from build123d import *

# Parameters (mm, degrees)
SKETCH_1_W      = 220
SKETCH_1_H      = 220
SKETCH_1_R      = 2
SKETCH_1_R_2    = 1.6
SKETCH_1_W_2    = 5
SKETCH_1_H_2    = 20
SKETCH_1_W_3    = 10
SKETCH_1_H_3    = 5.002557866
SKETCH_1_H_4    = 5
EXTRUDE_1_DEPTH = 5


with BuildPart() as part:
    # 草图1 → 凸台-拉伸1 (new body)
    with BuildSketch(Plane(origin=(0, 0, 0), x_dir=(0, 0, -1), z_dir=(1, 0, 0))):
        with Locations((1.240063593, -23.177255758)):
            Rectangle(SKETCH_1_W, SKETCH_1_H)
        with Locations((-22.759936407, 7.822744242)):
            Circle(SKETCH_1_R, mode=Mode.SUBTRACT)
        with Locations((-40.759936407, 7.822744242)):
            Circle(SKETCH_1_R, mode=Mode.SUBTRACT)
        with Locations((-40.759936407, 31.822744242)):
            Circle(SKETCH_1_R, mode=Mode.SUBTRACT)
        with Locations((-22.759936407, 31.822744242)):
            Circle(SKETCH_1_R, mode=Mode.SUBTRACT)
        with Locations((-22.759936407, -78.177255758)):
            Circle(SKETCH_1_R, mode=Mode.SUBTRACT)
        with Locations((-40.759936407, -78.177255758)):
            Circle(SKETCH_1_R, mode=Mode.SUBTRACT)
        with Locations((-40.759936407, -54.177255758)):
            Circle(SKETCH_1_R, mode=Mode.SUBTRACT)
        with Locations((-22.759936407, -54.177255758)):
            Circle(SKETCH_1_R, mode=Mode.SUBTRACT)
        with Locations((43.240063593, 7.822744242)):
            Circle(SKETCH_1_R, mode=Mode.SUBTRACT)
        with Locations((25.240063593, 7.822744242)):
            Circle(SKETCH_1_R, mode=Mode.SUBTRACT)
        with Locations((25.240063593, 31.822744242)):
            Circle(SKETCH_1_R, mode=Mode.SUBTRACT)
        with Locations((43.240063593, 31.822744242)):
            Circle(SKETCH_1_R, mode=Mode.SUBTRACT)
        with Locations((43.240063593, -78.177255758)):
            Circle(SKETCH_1_R, mode=Mode.SUBTRACT)
        with Locations((25.240063593, -78.177255758)):
            Circle(SKETCH_1_R, mode=Mode.SUBTRACT)
        with Locations((25.240063593, -54.177255758)):
            Circle(SKETCH_1_R, mode=Mode.SUBTRACT)
        with Locations((43.240063593, -54.177255758)):
            Circle(SKETCH_1_R, mode=Mode.SUBTRACT)
        with Locations((105.740063593, 81.322744242)):
            Circle(SKETCH_1_R_2, mode=Mode.SUBTRACT)
        with Locations((-103.259936407, 81.322744242)):
            Circle(SKETCH_1_R_2, mode=Mode.SUBTRACT)
        with Locations((-103.259936407, -127.677255758)):
            Circle(SKETCH_1_R_2, mode=Mode.SUBTRACT)
        with Locations((105.740063593, -127.677255758)):
            Circle(SKETCH_1_R_2, mode=Mode.SUBTRACT)
        with Locations((13.740063593, -23.177255758)):
            Rectangle(SKETCH_1_W_2, SKETCH_1_H_2, mode=Mode.SUBTRACT)
        with Locations((-11.259936407, -23.177255758)):
            Rectangle(SKETCH_1_W_2, SKETCH_1_H_2, mode=Mode.SUBTRACT)
        with Locations((1.240063593, -5.678534691)):
            Rectangle(SKETCH_1_W_3, SKETCH_1_H_3, mode=Mode.SUBTRACT)
        with Locations((1.240063593, -40.677255758)):
            Rectangle(SKETCH_1_W_3, SKETCH_1_H_4, mode=Mode.SUBTRACT)
    extrude(amount=EXTRUDE_1_DEPTH)


solid = part.part
Input: part model. Units: mm. Frame: model coordinates. A direction names the side the tool comes from. Coordinates: 2 decimals unless noted, no trailing zeros. Loops run counter-clockwise (first coordinate to the right, second up) from the corner with the lowest first, then second, coordinate; pieces in that order, holes last. Notation, with made-up numbers: (3.25, 70.25) -> (57.25, 70.25) arc R21 ccw to (57.25, 80.25) -> close; hole circle Ø5 at (-28, 57). An arc over 180 degrees is marked (long way). Write each question's results on one line, items separated by ' | '. Start each with the question number.
Q1. Section A-A, the plane y = -30.5. Return the cut outline in (x, z).
Q2. Section B-B, the plane z = -2. Return the cut outline in (x, y), plus the area to 3 significant figures.
Q3. Pin query (flat end, axial travel): pin 1 (3.5 mm diameter, centred on y = 31.82, z = 22.76, fed in from -X). Return the tip coordinate at first contact, or that it passes through.
Q4. Pull-direction query (Y, two-part tool) for faces 3 (the flat face through (2, 86.823, 0)), 4 (the flat face through (2, -23, 13.76)), 5 (the flat face through (2, -25, 108.76)); classes: released by +Y, released by -Y, zero draft, split by the parting line, or undercut.
Q5. Ray query, line 1 (Y direction, x = 2.4, z = -5.5); line 2 (Z direction, x = 4.35, y = -21.5); line 3 (Z direction, x = 4.85, y = -80). Return the intervals inside material, ascending. Write a range as from..to.
Q6. Reachability of faces 1 (the flat face through (0, -22, 0)), 2 (the flat face through (2, -38.177, -1)) from +Z, -Z, +X, -X, +Y, -Y: full face, straight path, thin tool, end or side. Return the list, or none.
Found:
1) outline: (0, -111.24) -> (5, -111.24) -> (5, -16.24) -> (0, -16.24) -> close; (0, -11.24) -> (5, -11.24) -> (5, 8.76) -> (0, 8.76) -> close; (0, 13.76) -> (5, 13.76) -> (5, 108.76) -> (0, 108.76) -> close
2) outline: (0, -133.18) -> (5, -133.18) -> (5, -43.18) -> (0, -43.18) -> close; (0, -38.18) -> (5, -38.18) -> (5, -8.18) -> (0, -8.18) -> close; (0, -3.18) -> (5, -3.18) -> (5, 86.82) -> (0, 86.82) -> close | area: 1,050 mm2
3) pin 1: through
4) face 3: released by +Y | face 4: undercut | face 5: zero draft
5) line 1: -133.18..-43.18, -38.18..-8.18, -3.18..86.82 | line 2: -111.24..-16.24, -11.24..8.76, 13.76..108.76 | line 3: -111.24..-44.06, -42.42..-26.06, -24.42..21.94, 23.58..39.94, 41.58..108.76
6) face 1: +Z, -Z, -X, +Y, -Y | face 2: +X, -X
